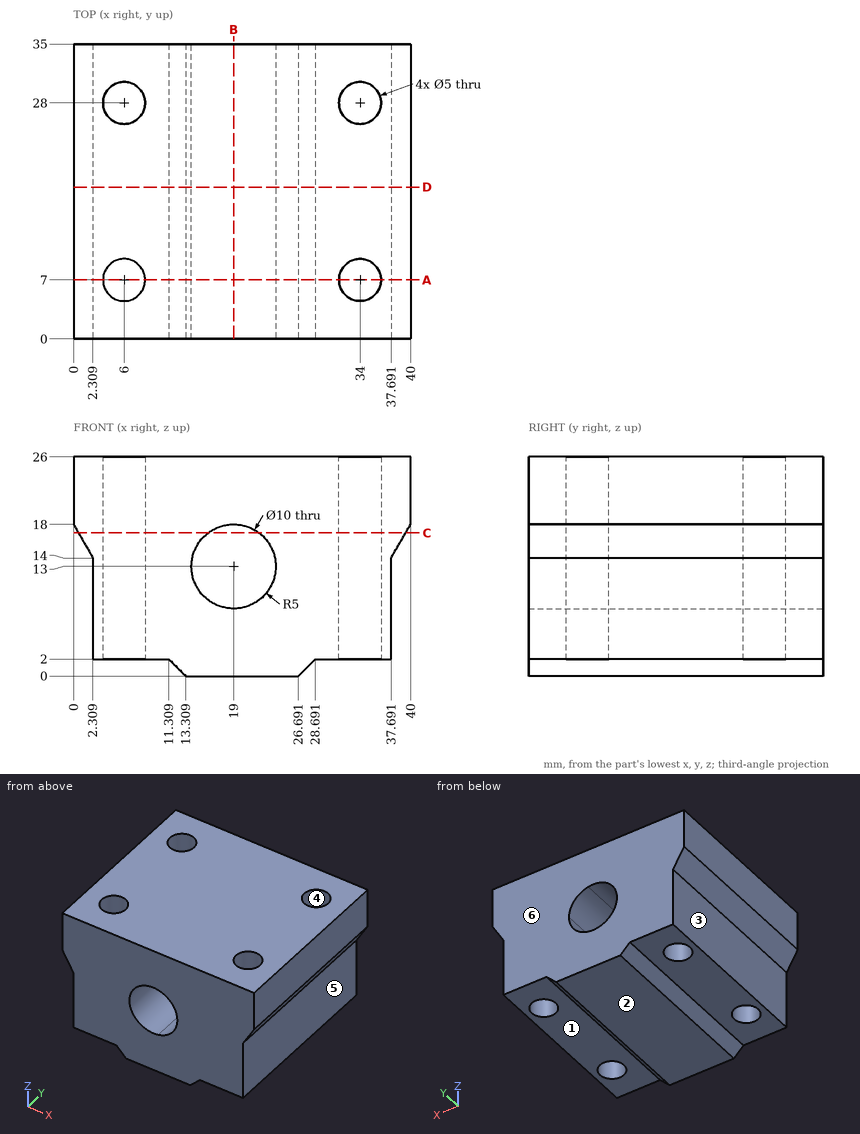
Could you check a few things on this drawing? It's one solid part, dimensions in mm from its lowest x, y, z. A direction names the side the tool comes from. Give positions to 0.01 mm unless a question says otherwise; leave off trailing zeros. Loops run counter-clockwise (first coordinate to the right, second up) from the corner with the lowest first, then second, coordinate; pieces in that order, holes last. Notation, with made-up numbers: M 87.5,41 L 95.5,41 A28 cw 95.5,70 Z; hole C 68.25,72.5 d5. An arc over 180 degrees is marked long. One line per question, with ' | ' between items. Start each with the question number.
Q1. If we mould it in two halves opening along Y, with no side actions, what happens to the marked faces 4, 5 and 6? For each: +Y half, -Y half, draft (parallel to the pull), parting line (faces both ways), or undercut.
Q2. If I drill on line 1 (X direction, y = 28, z = 19.5); line 2 (Y direction, x = 6, z = 11.5); line 3 (Z direction, x = 19, y = 13), over which ranges is the centre line in solid material (lowest first)? Write a range as from..to.
Q3. If we section it at A-A (y = 7): Please give me the cut outline in (x, z).
Q4. If we section it at D-D (y = 18): Please give me the cut outline in (x, z).
Q5. If we section it at B-B (x = 19): Please give me the cut outline in (y, z), plus the area to 3 significant figures.
Q6. If we section it at C-C (z = 17): Please give me the cut outline in (x, y), plus the area to 3 significant figures.
Q7. For the marked faces 1, 2 and 3, which set-ups out of +Z, -Z, +X, -X, +Y, -Y let a thin tool reach every point of the face, with its end or its side?
Q8. For pin 1 Ø4 at (x, y) = (6, 7) entering from +Z; pin 2 Ø6 at (x, y) = (6, 28) entering from -Z; pin 3 Ø6 at (y, z) = (30.5, 4) entering from +X; pin 4 Ø3.5 at (y, z) = (18, 7) entering from -X, each with a flat end and sliding along its axis, tell me the tip position at first contact or that it passes through.
Computed:
1) face 4: undercut | face 5: draft | face 6: +Y half
2) line 1: x = 0..3.5, 8.5..31.5, 36.5..40 | line 2: y = 0..4.5, 9.5..25.5, 30.5..35 | line 3: z = 0..8, 18..26
3) outline: M 0,18 L 2.31,14 L 2.31,2 L 3.5,2 L 3.5,26 L 0,26 Z; M 8.5,2 L 11.31,2 L 13.31,0 L 26.69,0 L 28.69,2 L 31.5,2 L 31.5,26 L 8.5,26 Z; M 36.5,2 L 37.69,2 L 37.69,14 L 40,18 L 40,26 L 36.5,26 Z; hole M 20,8.1 A5 ccw 20,17.9 A5 ccw long Z
4) outline: M 0,18 L 2.31,14 L 2.31,2 L 11.31,2 L 13.31,0 L 26.69,0 L 28.69,2 L 37.69,2 L 37.69,14 L 40,18 L 40,26 L 0,26 Z; hole M 20,8.1 A5 ccw 20,17.9 A5 ccw long Z
5) outline: M 0,0 L 35,0 L 35,8 L 0,8 Z; M 0,18 L 35,18 L 35,26 L 0,26 Z | area: 560 mm²
6) outline: M 0.58,0 L 16,0 L 16,35 L 0.58,35 Z; M 22,0 L 39.42,0 L 39.42,35 L 22,35 Z; hole C 6,7 d5; hole C 6,28 d5; hole C 34,7 d5; hole C 34,28 d5 | area: 1,070 mm²
7) face 1: -Z, +X, +Y, -Y | face 2: -Z, +X, -X, +Y, -Y | face 3: -Z, -X, +Y, -Y
8) pin 1: passes through | pin 2: stops at z = 2 | pin 3: stops at x = 37.69 | pin 4: stops at x = 2.31
